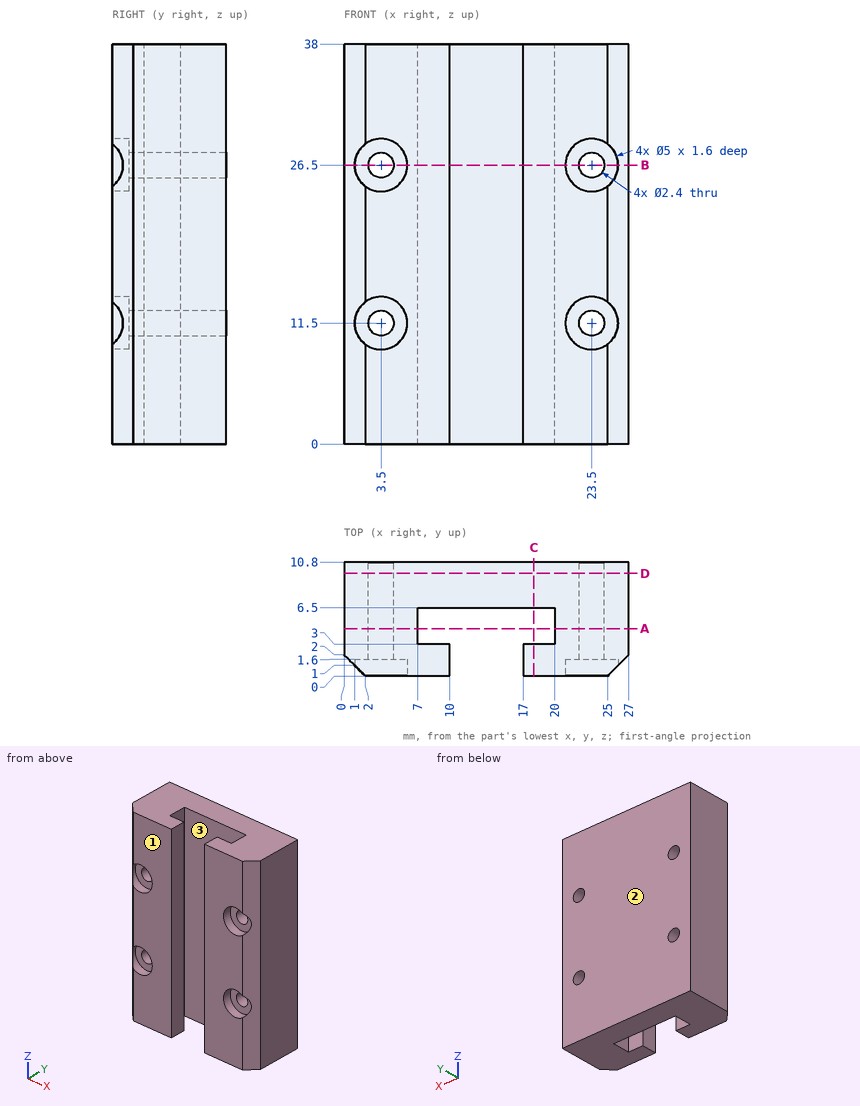
Input: dimensioned drawing with shaded views. Units: mm. Origin: part minimum x, y, z. Give positions to 0.01 mm unless a question says otherwise; leave off trailing zeros. Order: outer loops, then holes, each group sorted by start corner. A loop starts at its lowest first (then second) coordinate and runs counter-clockwise, first axis right, second up. Notation, with made-up numbers: (32.25, 60.25) -> (82.25, 60.25) arc R37 ccw to (82.25, 98.25) -> close; hole circle Ø7 at (-12, -36.75). An arc over 180 degrees is marked (long way). Use one line per item in the form item = value.
1) First-contact query: pin 1 Ø6 at (x, z) = (3.5, 11.5) entering from +Y; pin 2 Ø1.5 at (x, z) = (2.5, 11) entering from -Y. Flat tips, straight axial feed; report the tip coordinate or a pass-through.
Response values:
pin_1 = 10.8
pin_2 = 1.6
2) Section B-B, the plane z = 26.5. Return loops of the section in (x, y).
Response values:
outline = (0, 2) -> (1, 1) -> (1, 1.6) -> (2.3, 1.6) -> (2.3, 10.8) -> (0, 10.8) -> close; (4.7, 1.6) -> (6, 1.6) -> (6, 0) -> (10, 0) -> (10, 3) -> (7, 3) -> (7, 6.5) -> (20, 6.5) -> (20, 3) -> (17, 3) -> (17, 0) -> (21, 0) -> (21, 1.6) -> (22.3, 1.6) -> (22.3, 10.8) -> (4.7, 10.8) -> close; (24.7, 1.6) -> (26, 1.6) -> (26, 1) -> (27, 2) -> (27, 10.8) -> (24.7, 10.8) -> close
3) Section D-D, the plane y = 9.75. Return loops of the section in (x, z), and give its area (3 significant figures).
Response values:
outline = (0, 0) -> (27, 0) -> (27, 38) -> (0, 38) -> close; hole circle Ø2.4 at (3.5, 11.5); hole circle Ø2.4 at (3.5, 26.5); hole circle Ø2.4 at (23.5, 11.5); hole circle Ø2.4 at (23.5, 26.5)
area = 1,010 mm^2
4) Line query: probe 1 along X at (y, z) = (7.5, 26.5); probe 2 along Y at (x, z) = (7.5, 34.5); probe 3 along X at (y, z) = (3.75, 36.5). Output: solid intervals per line, ascending.
Response values:
probe_1 = 0 to 2.3, 4.7 to 22.3, 24.7 to 27
probe_2 = 0 to 3, 6.5 to 10.8
probe_3 = 0 to 7, 20 to 27
5) Section C-C, the plane x = 18. Return loops of the section in (y, z).
Response values:
outline = (0, 0) -> (3, 0) -> (3, 38) -> (0, 38) -> close; (6.5, 0) -> (10.8, 0) -> (10.8, 38) -> (6.5, 38) -> close
6) Section A-A, the plane y = 4.5. Return loops of the section in (x, z).
Response values:
outline = (0, 0) -> (7, 0) -> (7, 38) -> (0, 38) -> close; (20, 0) -> (27, 0) -> (27, 38) -> (20, 38) -> close; hole circle Ø2.4 at (3.5, 11.5); hole circle Ø2.4 at (3.5, 26.5); hole circle Ø2.4 at (23.5, 11.5); hole circle Ø2.4 at (23.5, 26.5)
7) Mould query, pull axis Y, two halves, no side actions, for the marked faces 1, 2 and 3. Classes: pulls with the +Y half, pulls with the -Y half, needs draft (parallel to the pull), parting line crosses it, or undercut.
Response values:
face_1 = pulls with the -Y half
face_2 = pulls with the +Y half
face_3 = undercut
